For this review, use the dimensioned drawing (mm, ordinates from the lowest corner) and the shaded views. Coordinates: 2 decimals unless noted, no trailing zeros. Order: outer loops, then holes, each group sorted by start corner. A loop starts at its lowest first (then second) coordinate and runs counter-clockwise, first axis right, second up. Notation, with made-up numbers: (2.5, 88) -> (54.5, 88) arc R12 cw to (54.5, 110) -> close; hole circle Ø5 at (39.5, 26.5). An arc over 180 degrees is marked (long way). Use one line per item in the form item = value. Start each with the question number.
(1) Insertion check: pin 1 Ø3 at (y, z) = (4, 6) entering from -X. The pin has a flat end and moves straight along its axis. Give the tip position at first contact, or say it passes through.
(2) Take a section at A-A (y = 2.1). State the section outline as (x, z) points, then the cut area to 3 significant figures.
(3) Take a section at B-B (z = 10). State the section outline as (x, y) points.
(4) Wall thickness on line 1 along X through (y, z) = (0.4, 7); line 2 along X through (y, z) = (2.7, 6): over which ranges is each line inside the solid? List them lowest first.
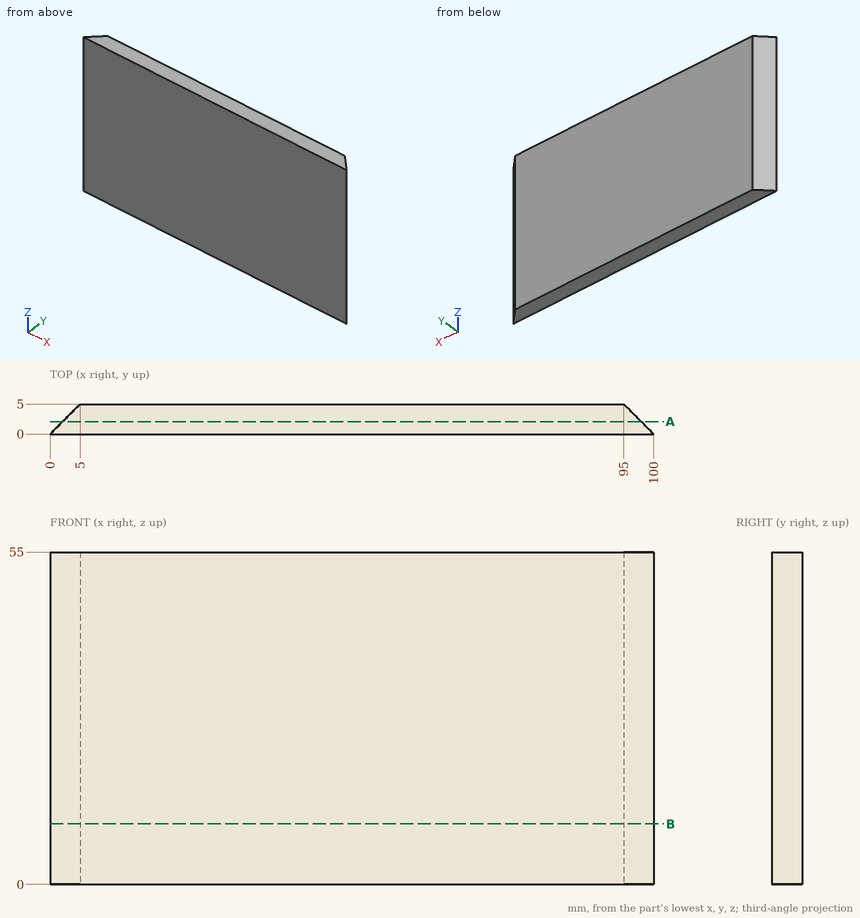
Findings:
q1.pin_1 = 2.5
q2.outline = (2.1, 0) -> (97.9, 0) -> (97.9, 55) -> (2.1, 55) -> close
q2.area = 5,270 mm²
q3.outline = (0, 0) -> (100, 0) -> (95, 5) -> (5, 5) -> close
q4.line_1 = 0.4 to 99.6
q4.line_2 = 2.7 to 97.3
